The drawing under review shows one solid part. Ordinate dimensions are in mm from its lowest x, y, z. A direction names the side the tool comes from. Coordinates: 2 decimals unless noted, no trailing zeros. Order: outer loops, then holes, each group sorted by start corner. A loop starts at its lowest first (then second) coordinate and runs counter-clockwise, first axis right, second up.
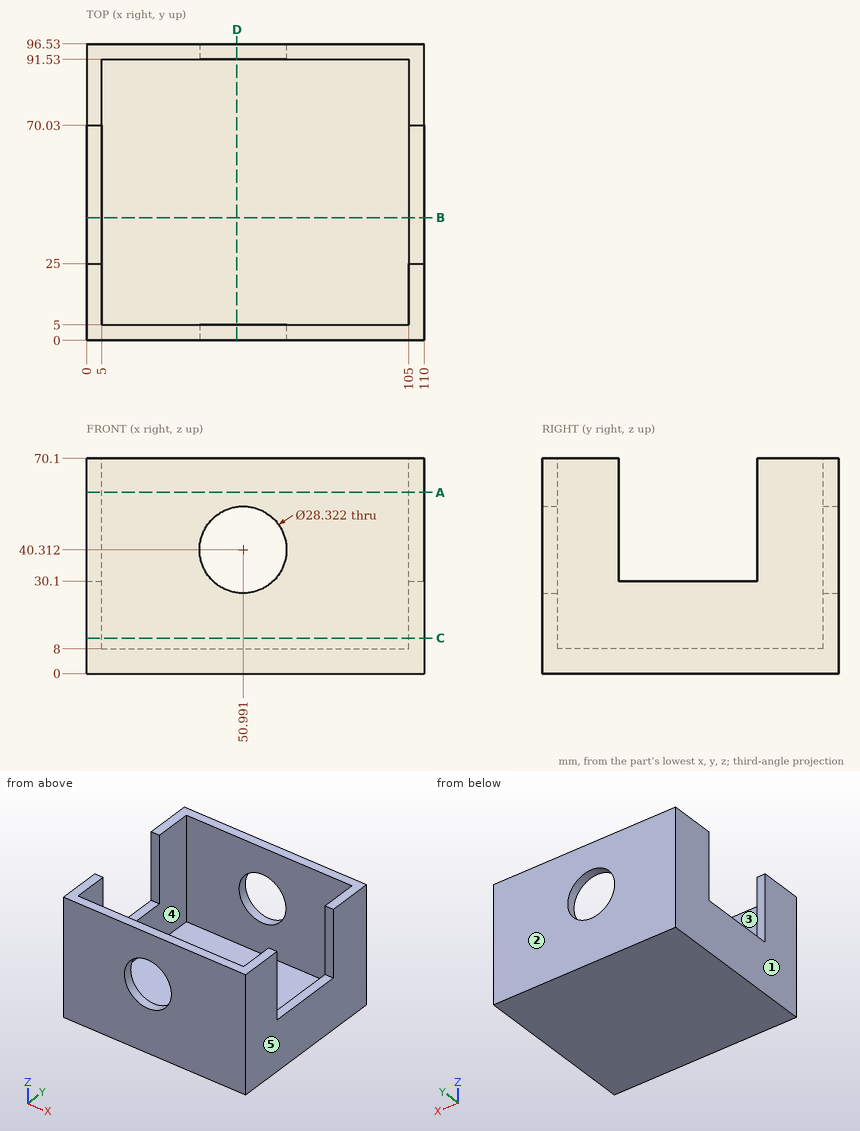
(1) Consider section A-A (z = 59). Give the boundary of the cut face in (x, y).
(2) Insertion check: pin 1 Ø4 at (x, y) = (1.5, 37.5) entering from +Z. The pin has a flat end and moves straight along its axis. Give the tip position at first contact, or say it passes through.
(3) Consider section B-B (y = 40). Give the boundary of the cut face in (x, z), then the cut area to 3 significant figures.
(4) Wall thickness on line 1 (Y direction, x = 72, z = 11); line 2 (X direction, y = 55.5, z = 25.5); line 3 (Z direction, x = 96.5, y = 76.5): over which ranges is each line inside the solid? List them lowest first.
(5) Consider section C-C (z = 11.5). Give the boundary of the cut face in (x, y).
(6) Consider section D-D (x = 49). Give the boundary of the cut face in (y, z).
(7) The part is to be moulded in two halves that separate along Y. For the marked faces 1, 2 and 3, say which applies: +Y half, -Y half, draft (parallel to the pull), parting line (faces both ways), or undercut.
(8) Tool access review of the marked faces 4 and 5: name each direction out of +Z, -Z, +X, -X, +Y, -Y from which nothing blocks a thin tool from reaching the whole face with its end or side.
Findings:
1. outline: (0, 0) - (110, 0) - (110, 25) - (105, 25) - (105, 5) - (5, 5) - (5, 25) - (0, 25) - close; (0, 70.03) - (5, 70.03) - (5, 91.53) - (105, 91.53) - (105, 70.03) - (110, 70.03) - (110, 96.53) - (0, 96.53) - close
2. pin 1: stops at z = 30.1
3. outline: (0, 0) - (110, 0) - (110, 30.1) - (105, 30.1) - (105, 8) - (5, 8) - (5, 30.1) - (0, 30.1) - close
3. area: 1,100 mm2
4. line 1: y = 0 to 5, 91.53 to 96.53
4. line 2: x = 0 to 5, 105 to 110
4. line 3: z = 0 to 8
5. outline: (0, 0) - (110, 0) - (110, 96.53) - (0, 96.53) - close; hole (5, 5) - (105, 5) - (105, 91.53) - (5, 91.53) - close
6. outline: (0, 0) - (96.53, 0) - (96.53, 26.29) - (91.53, 26.29) - (91.53, 8) - (5, 8) - (5, 26.29) - (0, 26.29) - close; (0, 54.33) - (5, 54.33) - (5, 70.1) - (0, 70.1) - close; (91.53, 54.33) - (96.53, 54.33) - (96.53, 70.1) - (91.53, 70.1) - close
7. face 1: draft
7. face 2: +Y half
7. face 3: undercut
8. face 4: +Z
8. face 5: +Z, -Z, +X, +Y, -Y
